from build123d import *

# Parameters (mm, degrees)
SKETCH_1_R          = 55
EXTRUDE_1_DEPTH     = 3
SKETCH_3_R          = 1.65
CUT_EXTRUDE_1_DEPTH = 3
CUT_EXTRUDE_2_DEPTH = 3
SKETCH_5_R          = 6.5
CUT_EXTRUDE_3_DEPTH = 3


with BuildPart() as part:
    # 草图1 → 凸台-拉伸1 (new body)
    with BuildSketch(Plane.XY):
        Circle(SKETCH_1_R)
    extrude(amount=EXTRUDE_1_DEPTH)

    # 草图3 → 切除-拉伸1 (cut)
    with BuildSketch(Plane.XY.offset(3)):
        with Locations((27.5, 35)):
            Circle(SKETCH_3_R)
        with Locations((-27.5, 35)):
            Circle(SKETCH_3_R)
    extrude(amount=-CUT_EXTRUDE_1_DEPTH, mode=Mode.SUBTRACT)

    # 草图4 → 切除-拉伸2 (cut)
    with BuildSketch(Plane.XY.offset(3)):
        with BuildLine():
            ThreePointArc((15.073713466, 11.566467151), (17.553711118, 7.270985215), (18.837452366, 2.479997652))
            Line((18.837452366, 2.479997652), (39.657794455, 5.221047689))
            ThreePointArc((39.657794455, 5.221047689), (36.9551813, 15.307337295), (31.734133612, 24.35045716))
            Line((31.734133612, 24.35045716), (15.073713466, 11.566467151))
        make_face()
        with BuildLine():
            Line((-39.657794455, 5.221047689), (-18.837452366, 2.479997652))
            ThreePointArc((-18.837452366, 2.479997652), (-17.553711118, 7.270985215), (-15.073713466, 11.566467151))
            Line((-15.073713466, 11.566467151), (-31.734133612, 24.35045716))
            ThreePointArc((-31.734133612, 24.35045716), (-36.9551813, 15.307337295), (-39.657794455, 5.221047689))
        make_face()
        with BuildLine():
            Line((-31.734133612, -24.35045716), (-15.073713466, -11.566467151))
            ThreePointArc((-15.073713466, -11.566467151), (-17.553711118, -7.270985215), (-18.837452366, -2.479997652))
            Line((-18.837452366, -2.479997652), (-39.657794455, -5.221047689))
            ThreePointArc((-39.657794455, -5.221047689), (-36.9551813, -15.307337295), (-31.734133612, -24.35045716))
        make_face()
        with BuildLine():
            Line((-5.221047689, -39.657794455), (-2.479997652, -18.837452366))
            ThreePointArc((-2.479997652, -18.837452366), (-7.270985215, -17.553711118), (-11.566467151, -15.073713466))
            Line((-11.566467151, -15.073713466), (-24.35045716, -31.734133612))
            ThreePointArc((-24.35045716, -31.734133612), (-15.307337295, -36.9551813), (-5.221047689, -39.657794455))
        make_face()
        with BuildLine():
            Line((24.35045716, -31.734133612), (11.566467151, -15.073713466))
            ThreePointArc((11.566467151, -15.073713466), (7.270985215, -17.553711118), (2.479997652, -18.837452366))
            Line((2.479997652, -18.837452366), (5.221047689, -39.657794455))
            ThreePointArc((5.221047689, -39.657794455), (15.307337295, -36.9551813), (24.35045716, -31.734133612))
        make_face()
        with BuildLine():
            Line((39.657794455, -5.221047689), (18.837452366, -2.479997652))
            ThreePointArc((18.837452366, -2.479997652), (17.553711118, -7.270985215), (15.073713466, -11.566467151))
            Line((15.073713466, -11.566467151), (31.734133612, -24.35045716))
            ThreePointArc((31.734133612, -24.35045716), (36.9551813, -15.307337295), (39.657794455, -5.221047689))
        make_face()
    extrude(amount=-CUT_EXTRUDE_2_DEPTH, mode=Mode.SUBTRACT)

    # 草图5 → 切除-拉伸3 (cut)
    with BuildSketch(Plane.XY.offset(3)):
        Circle(SKETCH_5_R)
    extrude(amount=-CUT_EXTRUDE_3_DEPTH, mode=Mode.SUBTRACT)


solid = part.part
Could you check a few things on this model? Use its own coordinates, in mm. A direction names the side the tool comes from. Give positions to 0.01 mm unless a question says otherwise; leave off trailing zeros. Order: outer loops, then holes, each group sorted by start corner. A loop starts at its lowest first (then second) coordinate and runs counter-clockwise, first axis right, second up. Notation, with made-up numbers: (-5, 61.25) -> (32, 61.25) arc R13 cw to (32, 86.25) -> close; hole circle Ø5 at (24, 70.5). An arc over 180 degrees is marked (long way). Return JSON: item names as keys, results as strings.
1. I need wall thicknesses on line 1 (Y direction, x = -27.5, z = 2.2); line 2 (X direction, y = -20.5, z = 2.15); line 3 (Y direction, x = 0, z = 1). Which ranges of each line are inside material? Lowest first, please. Write a range as from..to.
Answer list:
{"line 1": "y = -47.63..-21.1, -3.62..3.62, 21.1..33.35, 36.65..47.63", "line 2": "x = -51.04..-34.35, -26.72..-15.73, -2.7..2.7, 15.73..26.72, 34.35..51.04", "line 3": "y = -55..-6.5, 6.5..55"}
2. Imagine slicing it at A-A on x = 0. List the corners of the cut face in (y, z) for me.
Answer list:
{"outline": "(-55, 0) -> (-6.5, 0) -> (-6.5, 3) -> (-55, 3) -> close; (6.5, 0) -> (55, 0) -> (55, 3) -> (6.5, 3) -> close"}
3. Imagine slicing it at C-C on z = 2.5. Give the number of separate pieces and of enclosed holes in the cut face, then the cut area to 3 significant figures.
Answer list:
{"separate pieces": "1", "enclosed holes": "9", "area": "7,410 mm2"}
4. On a 3-axis mill with a long thin cutter (end or side, diameter ignored), from which of +Z, -Z, +X, -X, +Y, -Y can I reach the whole of each face in a straight line? I mean faces 1 (the flat face through (11, 1, 0)), 2 (the cylindrical face through (36.9, -15.44, 1.52)). Say none if no direction works.
Answer list:
{"face 1": "-Z, +X, -X, +Y, -Y", "face 2": "+Z, -Z"}
5. Imagine slicing it at B-B on y = 35. List the corners of the cut face in (x, z) for me, then the cut area to 3 significant figures.
Answer list:
{"outline": "(-42.43, 0) -> (-29.15, 0) -> (-29.15, 3) -> (-42.43, 3) -> close; (-25.85, 0) -> (25.85, 0) -> (25.85, 3) -> (-25.85, 3) -> close; (29.15, 0) -> (42.43, 0) -> (42.43, 3) -> (29.15, 3) -> close", "area": "235 mm2"}
6. For pin 1 Ø3 at (x, y) = (-13.5, -0.5) entering from -Z; pin 2 Ø1 at (x, z) = (-44, 1.5) entering from +Y; pin 3 Ø4 at (x, y) = (1, 3.5) entering from -Z; pin 4 Ø1.5 at (x, z) = (-32, 1.5) entering from -Y, each with a flat end and sliding along its axis, tell me the tip position at first contact or that it passes through.
Answer list:
{"pin 1": "stops at z = 0", "pin 2": "stops at y = 33.66", "pin 3": "passes through", "pin 4": "stops at y = -45.26"}
